Can you work these out from the model? Positions are in its coordinate system, mm. Face numbers are marked on the shaded views. Coordinates: 2 decimals unless noted, no trailing zeros. Write each loop counter-clockwise with the first axis right and the second up, starting at its lowest first coordinate (ties: lowest second). Pieces come first, ordered by that corner, then holes.
```python
from build123d import *

# Parameters (mm, degrees)
F1_DEPTH = 40.1828
F2_W     = 2.54
F2_H     = 17.78
F5_R     = 2.667
F6_DEPTH = 25.4
F8_R     = 5.715
F9_DEPTH = 25.4


with BuildPart() as f1:
    # F0 (on Front) → F1 (new body)
    with BuildSketch(Plane.XZ):
        with BuildLine():
            Line((-50.8, 0), (50.8, 0))
            Line((50.8, 0), (50.8, 15.875))
            Line((50.8, 15.875), (50.8, 31.75))
            Line((50.8, 31.75), (35.305086, 31.75))
            ThreePointArc((35.305086, 31.75), (0, 12.7), (-35.305086, 31.75))
            Line((-35.305086, 31.75), (-50.8, 31.75))
            Line((-50.8, 31.75), (-50.8, 15.875))
            Line((-50.8, 15.875), (-50.8, 0))
        make_face()
        Polygon((-73.025, 0), (-50.8, 0), (-50.8, 15.875), (-73.025, 3.578278), align=None)
        Polygon((50.8, 15.875), (50.8, 0), (73.025, 0), (73.025, 3.578278), align=None)
    extrude(amount=F1_DEPTH)

    # F2 (on face) → F4 (revolve, cut)
    with BuildSketch(Plane.XY.offset(31.75)):
        with Locations((-43.052543, -20.0914)):
            Rectangle(F2_W, F2_H)
    revolve(axis=Axis((0, -22.422592, 54.9402), (0, -1, 0)), mode=Mode.SUBTRACT)

    # F5 (on Top) → F6 (cut)
    with BuildSketch(Plane.XY):
        with Locations((-60.325, -30.1371)):
            Circle(F5_R)
        with Locations((-60.325, -10.0457)):
            Circle(F5_R)
        with Locations((60.325, -30.1371)):
            Circle(F5_R)
        with Locations((60.325, -10.0457)):
            Circle(F5_R)
    extrude(amount=F6_DEPTH, mode=Mode.SUBTRACT)

    # F8 (on offset) → F9 (cut)
    with BuildSketch(Plane.XY.offset(7.62)):
        with Locations((60.325, -30.1371)):
            Circle(F8_R)
        with Locations((60.325, -10.0457)):
            Circle(F8_R)
        with Locations((-60.325, -30.1371)):
            Circle(F8_R)
        with Locations((-60.325, -10.0457)):
            Circle(F8_R)
    extrude(amount=F9_DEPTH, mode=Mode.SUBTRACT)


solid = f1.part
```
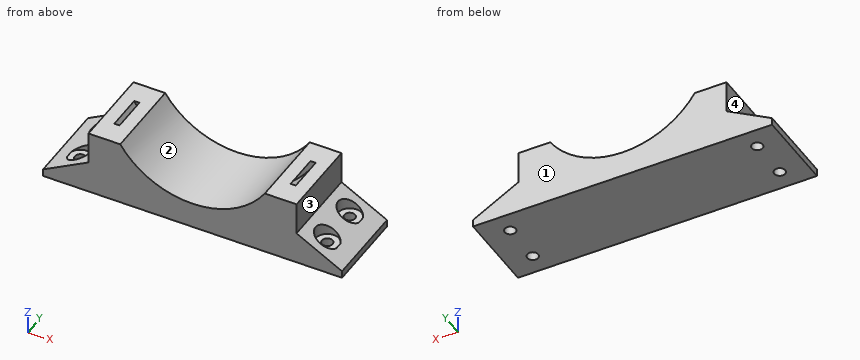
1. If we section it at B-B, the plane y = -23: List the corners of the cut face in (x, z) for me (3 decimals).
2. We'd pull the mould along X, two halves only. Please class the marked faces 1, 2, 3 and 4: released by +X, released by -X, zero draft, split by the parting line, or undercut.
3. If we section it at A-A, the plane z = 24: List the corners of the cut face in (x, y) for me, plus the area to 3 significant figures.
4. I'm going to push flat-ended pins straight in: P1, Ø5.5, axis at x = 57.5, y = -30, coming from the +Z side; P2, Ø4, axis at x = 53, z = 27, coming from the +Y side; P3, Ø8, axis at y = -11, z = 23, coming from the +X side; P4, Ø12, axis at x = -61, y = -12.5, coming from the +Z side. Where does each tip first touch, or does it pass through?
5. If we section it at C-C, the plane z = 10.5: List the corners of the cut face in (x, y) for me (3 decimals), plus the area to 3 significant figures.
6. If I drill on L1, parallel to X at y = -11.5, z = 23; L2, parallel to X at y = -24, z = 24; L3, parallel to Y at x = -33, z = 18, over which ranges is the centre line in solid material (lowest first)?
7. If we section it at D-D, the plane y = -14: List the corners of the cut face in (x, z) for me (3 decimals), plus the area to 3 significant figures.
Answers:
1. outline: (-73.025, 0) - (73.025, 0) - (73.025, 3.578) - (50.8, 15.875) - (50.8, 31.75) - (44.323, 31.75) arc R50.023 cw to (-44.323, 31.75) - (-50.8, 31.75) - (-50.8, 15.875) - (-73.025, 3.578) - close; (-41.783, 31.75) arc R47.787 ccw to (41.783, 31.75) - (35.305, 31.75) arc R42.24 cw to (-35.305, 31.75) - close
2. face 1: zero draft
2. face 2: undercut
2. face 3: released by +X
2. face 4: released by -X
3. outline: (-50.8, -40.18) - (-28.76, -40.18) - (-28.76, 0) - (-50.8, 0) - close; (28.76, -40.18) - (50.8, -40.18) - (50.8, 0) - (28.76, 0) - close; hole (-39.31, -28.98) - (-36.42, -28.98) - (-36.42, -11.2) - (-39.31, -11.2) - close; hole (36.42, -28.98) - (39.31, -28.98) - (39.31, -11.2) - (36.42, -11.2) - close
3. area: 1,670 mm2
4. P1: stops at z = 7.62
4. P2: passes through
4. P3: stops at x = 50.8
4. P4: stops at z = 13.55
5. outline: (-60.515, -40.183) - (60.515, -40.183) - (60.515, -35.849) arc R5.715 cw (long way) to (60.515, -24.425) - (60.515, -15.758) arc R5.715 cw (long way) to (60.515, -4.334) - (60.515, 0) - (-60.515, 0) - (-60.515, -4.334) arc R5.715 cw (long way) to (-60.515, -15.758) - (-60.515, -24.425) arc R5.715 cw (long way) to (-60.515, -35.849) - close; hole (-22.964, -28.981) - (-17.568, -28.981) - (-17.568, -11.201) - (-22.964, -11.201) - close; hole (17.568, -28.981) - (22.964, -28.981) - (22.964, -11.201) - (17.568, -11.201) - close
5. area: 4,460 mm2
6. L1: x = -50.8 to -38.5, -35.54 to -27.64, 27.64 to 35.54, 38.5 to 50.8
6. L2: x = -50.8 to -39.31, -36.42 to -28.76, 28.76 to 36.42, 39.31 to 50.8
6. L3: y = -40.18 to -28.98, -11.2 to 0
7. outline: (-73.025, 0) - (73.025, 0) - (73.025, 3.578) - (64.451, 8.322) - (64.451, 7.62) - (56.199, 7.62) - (56.199, 12.888) - (50.8, 15.875) - (50.8, 31.75) - (44.323, 31.75) arc R50.023 cw to (-44.323, 31.75) - (-50.8, 31.75) - (-50.8, 15.875) - (-56.199, 12.888) - (-56.199, 7.62) - (-64.451, 7.62) - (-64.451, 8.322) - (-73.025, 3.578) - close; (-41.783, 31.75) arc R47.787 ccw to (41.783, 31.75) - (35.305, 31.75) arc R42.24 cw to (-35.305, 31.75) - close
7. area: 2,430 mm2
